Autodesk Inventor part; units mm, degrees
ref_plane "YZ Plane" through (0, 0, 0) normal (1, 0, 0) x (0, 1, 0)
ref_plane "XZ Plane" through (0, 0, 0) normal (0, 1, 0) x (-1, 0, 0)
ref_plane "XY Plane" through (0, 0, 0) normal (0, 0, 1) x (1, 0, 0)
sketch "Sketch1" plane through (0, 0, 0) normal (0, 1, 0) x (-1, 0, 0)
  line L0 (15.2617, 5.412) -> (-15.7383, 36.412) construction
  line L1 (15.2617, 36.412) -> (-15.7383, 5.412) construction
  line L2 (48.4032, 51.2455) -> (-48.8799, 51.2455) construction
  line L3 (-48.8799, 51.2455) -> (-48.8799, 71.2455) construction
  line L4 (-48.8799, 71.2455) -> (48.4032, 71.2455) construction
  line L5 (48.4032, 71.2455) -> (48.4032, 51.2455) construction
  line L6 (48.4032, 51.2455) -> (-48.8799, 71.2455) construction
  line L7 (-48.8799, 51.2455) -> (48.4032, 71.2455) construction
  line L8 (16.9077, -0.088) -> (-17.3843, -0.088)
  line L9 (-21.2383, 3.766) -> (-21.2383, 38.058)
  line L10 (-17.3843, 41.912) -> (16.9077, 41.912)
  line L11 (20.7617, 38.058) -> (20.7617, 3.766)
  line L12 (20.7617, -0.088) -> (-21.2383, 41.912) construction
  line L13 (-21.2383, -0.088) -> (20.7617, 41.912) construction
  line L14 (20.7617, 3.766) -> (16.9077, -0.088)
  line L15 (-17.3843, -0.088) -> (-21.2383, 3.766)
  line L16 (-17.3843, 41.912) -> (-21.2383, 38.058)
  line L17 (16.9077, 41.912) -> (20.7617, 38.058)
  circle A0 centre (36.4032, 39.2455) radius 12 construction
  circle A1 centre (-36.8799, 39.2455) radius 12 construction
  circle A2 centre (-0.0151, 83.2455) radius 12 construction
  line L18 (-0.2367, 13.9012) -> (-0.24, 27.9229) construction
  line L19 (7.7643, 13.9031) -> (7.761, 27.9248)
  line L20 (-8.241, 27.921) -> (-8.2377, 13.8992)
  arc A3 (-8.2377, 13.8992) -> (7.7643, 13.9031) centre (-0.2367, 13.9012) ccw
  arc A4 (7.761, 27.9248) -> (-8.241, 27.921) centre (-0.24, 27.9229) ccw
  line L21 (36.4032, 35.4355) -> (36.4032, 43.0555) construction
  line L22 (39.1532, 35.4355) -> (39.1532, 43.0555)
  line L23 (33.6532, 43.0555) -> (33.6532, 35.4355)
  arc A5 (33.6532, 35.4355) -> (39.1532, 35.4355) centre (36.4032, 35.4355) ccw
  arc A6 (39.1532, 43.0555) -> (33.6532, 43.0555) centre (36.4032, 43.0555) ccw
  line L24 (-36.8799, 35.4355) -> (-36.8799, 43.0555) construction
  line L25 (-34.1299, 35.4355) -> (-34.1299, 43.0555)
  line L26 (-39.6299, 43.0555) -> (-39.6299, 35.4355)
  arc A7 (-39.6299, 35.4355) -> (-34.1299, 35.4355) centre (-36.8799, 35.4355) ccw
  arc A8 (-34.1299, 43.0555) -> (-39.6299, 43.0555) centre (-36.8799, 43.0555) ccw
  line L27 (-0.0151, 79.4355) -> (-0.0151, 87.0555) construction
  line L28 (2.7349, 79.4355) -> (2.7349, 87.0555)
  line L29 (-2.7651, 87.0555) -> (-2.7651, 79.4355)
  arc A9 (-2.7651, 79.4355) -> (2.7349, 79.4355) centre (-0.0151, 79.4355) ccw
  arc A10 (2.7349, 87.0555) -> (-2.7651, 87.0555) centre (-0.0151, 87.0555) ccw
  ellipse E0 centre (-0.2383, 39.985) end of major axis (-0.2383, 96.6561) minor radius 44.4552
  circle A11 centre (15.2617, 5.412) radius 1.5
  circle A12 centre (-15.7383, 5.412) radius 1.5
  circle A13 centre (-15.7383, 36.412) radius 1.5
  circle A14 centre (15.2617, 36.412) radius 1.5
  circle A15 centre (-0.2383, 20.912) radius 12.5
  point P0 (-0.2383, 61.2455)
  point P1 (-0.2383, 61.2455)
  point P2 (-0.2383, 20.912)
  point P3 (7.1468, 30.9972)
  point P4 (7.1516, 10.8304)
  point P5 (-7.6234, 10.8269)
  point P6 (-7.6283, 30.9936)
  dimension "d45" = 31
  dimension "d46" = 31
  dimension "d47" = 20
  dimension "d48" = 12
  dimension "d49" = 12
  dimension "d50" = 42
  dimension "d51" = 42
  dimension "d52" = 3.854
  dimension "d53" = 45
  dimension "d54" = 3.854
  dimension "d55" = 45
  dimension "d56" = 3.854
  dimension "d57" = 45
  dimension "d58" = 3.854
  dimension "d59" = 45
  dimension "d60" = 12
  dimension "d61" = 16.002
  dimension "d63" = 3.81
  dimension "d64" = 5.5
  dimension "d65" = 3.81
  dimension "d66" = 5.5
  dimension "d67" = 3.81
  dimension "d68" = 5.5
  dimension "d71" = 3
  dimension "d72" = 3
  dimension "d73" = 3
  dimension "d74" = 3
  dimension "d75" = 25
extrude "Extrusion4" add sketch "Sketch1" along normal blind 5 contours L8 L15 L9 L16 L10 L17 L11 L14 | E0
equation "\"d54\" = d52"
equation "\"d56\" = d54"
equation "\"d57\" = d55"
equation "\"d58\" = d54"
equation "\"d59\" = d55"
equation "\"d65\" = d63"
equation "\"d66\" = d64"
equation "\"d67\" = d65"
equation "\"d68\" = d64"
equation "\"d72\" = d71"
equation "\"d73\" = d72"
equation "\"d74\" = d73"
properties part number "Base Plate" material "Acrylic"
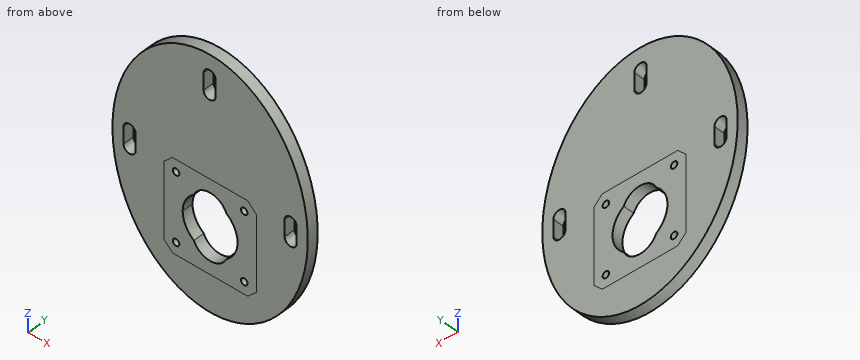
Geometry check sheet. Reference: the model listing, model coordinates, mm. Round coordinates to 2 decimals unless told otherwise and drop trailing zeros. Use a Markdown table: item, result.
Q1. Cross-section at A-A on y = 2.45. State how many separate pieces and enclosed holes the cut face has, plus the area to 3 significant figures.
Solutions:
| item | result |
|---|---|
| separate pieces | 1 |
| enclosed holes | 8 |
| area | 7,140 mm2 |
Q2. Go/stop test with flat-tipped pins: P1, Ø1.5, axis at y = 2.5, z = 83.5, coming from the +X side; P2, Ø2.5, axis at x = -15.26, z = 5.41, coming from the +Y side; P3, Ø2, axis at x = 16, y = 3.5, coming from the +Z side; P4, Ø2.5, axis at y = 3.5, z = 38, coming from the -X side. Record where each tip stops, or that it passes through.
Solutions:
| item | result |
|---|---|
| P1 | stops at x = 29.41 |
| P2 | passes through |
| P3 | stops at z = 93.44 |
| P4 | stops at x = -44.21 |
Q3. Material ranges on line 1 (X direction, y = 3.45, z = 39); line 2 (Z direction, x = -1, y = 2.85); line 3 (X direction, y = 3.7, z = 43.5), recorded low to high.
Solutions:
| item | result |
|---|---|
| line 1 | x = -44.21 to -39.15, -33.65 to 34.13, 39.63 to 44.69 |
| line 2 | z = -16.66 to 6, 35.83 to 76.88, 89.61 to 96.63 |
| line 3 | x = -44.13 to -39.12, -33.69 to 34.17, 39.59 to 44.61 |
